Check sheet for the drawn part. Datum: minimum x, y, z corner. Units: mm. A direction names the side the tool comes from. Coordinates: 2 decimals unless noted, no trailing zeros. Write each loop counter-clockwise with the first axis right and the second up, starting at its lowest first coordinate (ties: lowest second). Pieces come first, ordered by that corner, then holes. Notation, with made-up numbers: (9, -39.5) -> (18, -39.5) arc R28 ccw to (18, -18.5) -> close; hole circle Ø4 at (29.25, 88). An arc over 180 degrees is marked (long way). Answer in a Markdown table with one row per item.
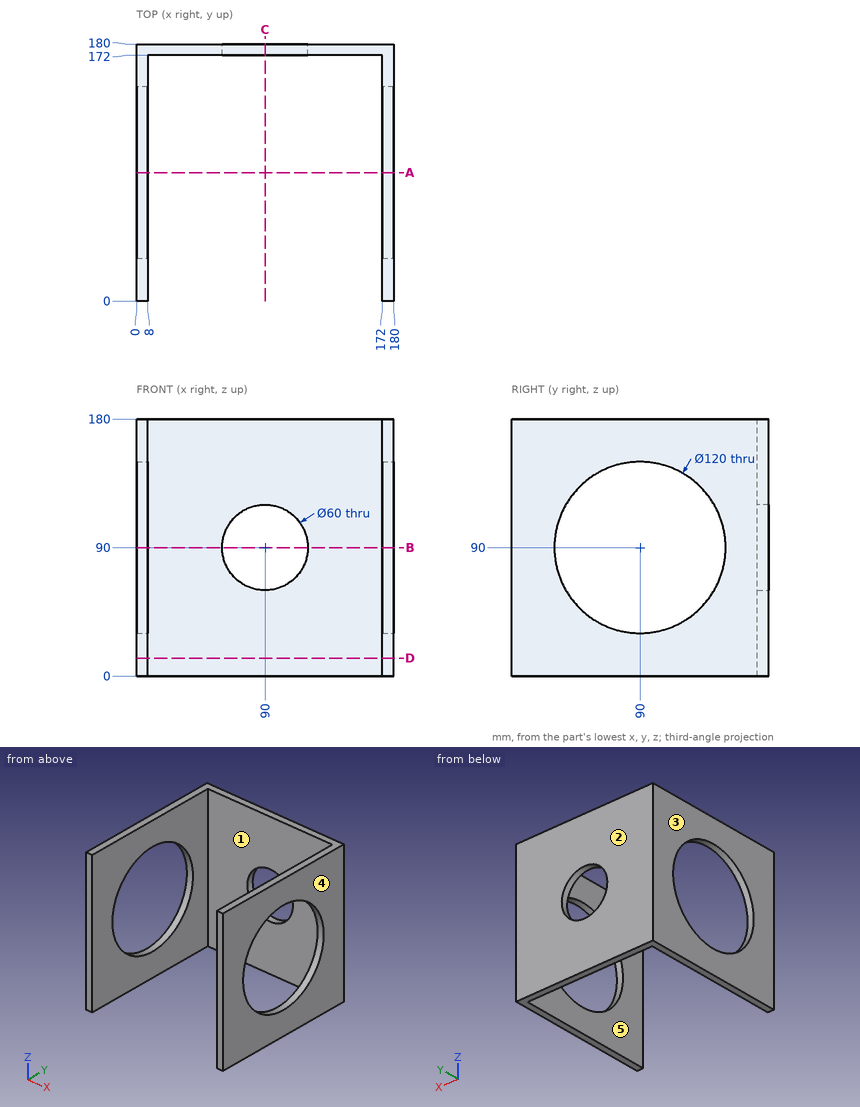
1. Sectioned sample at C-C, the plane x = 90. Record the cut outline in (y, z), and give its area (3 significant figures).
Findings below:
| item | result |
|---|---|
| outline | (172, 0) -> (180, 0) -> (180, 60) -> (172, 60) -> close; (172, 120) -> (180, 120) -> (180, 180) -> (172, 180) -> close |
| area | 960 mm² |
2. Material ranges on probe 1 along Z at (x, y) = (3, 90); probe 2 along X at (y, z) = (10.5, 97.5); probe 3 along Y at (x, z) = (34, 145.5), recorded low to high. Write a range as from..to.
Findings below:
| item | result |
|---|---|
| probe 1 | z = 0..30, 150..180 |
| probe 2 | x = 0..8, 172..180 |
| probe 3 | y = 172..180 |
3. Go/stop test with a flat-tipped pin: pin 1 (2 mm diameter, centred on x = 141, z = 111, fed in from -Y). Record where the tip stops, or that it passes through.
Findings below:
| item | result |
|---|---|
| pin 1 | stops at y = 172 |
4. Access from +Z, -Z, +X, -X, +Y, -Y to the whole of each face (thin tool, end or side, straight path). Record for the marked faces 1 and 2.
Findings below:
| item | result |
|---|---|
| face 1 | +Z, -Z, -Y |
| face 2 | +Z, -Z, +X, -X, +Y |
5. Sectioned sample at D-D, the plane z = 12.5. Record the cut outline in (x, y).
Findings below:
| item | result |
|---|---|
| outline | (0, 0) -> (8, 0) -> (8, 172) -> (172, 172) -> (172, 0) -> (180, 0) -> (180, 180) -> (0, 180) -> close |
6. Release check for a two-part mould opening along X. For the marked faces 3, 4 and 5 record: released by +X, released by -X, zero draft, split by the parting line, or undercut.
Findings below:
| item | result |
|---|---|
| face 3 | released by -X |
| face 4 | released by +X |
| face 5 | undercut |
7. Sectioned sample at A-A, the plane y = 90. Record the cut outline in (x, z), and give its area (3 significant figures).
Findings below:
| item | result |
|---|---|
| outline | (0, 0) -> (8, 0) -> (8, 30) -> (0, 30) -> close; (0, 150) -> (8, 150) -> (8, 180) -> (0, 180) -> close; (172, 0) -> (180, 0) -> (180, 30) -> (172, 30) -> close; (172, 150) -> (180, 150) -> (180, 180) -> (172, 180) -> close |
| area | 960 mm² |
8. Sectioned sample at B-B, the plane z = 90. Record the cut outline in (x, y), and give its area (3 significant figures).
Findings below:
| item | result |
|---|---|
| outline | (0, 0) -> (8, 0) -> (8, 30) -> (0, 30) -> close; (0, 150) -> (8, 150) -> (8, 172) -> (60, 172) -> (60, 180) -> (0, 180) -> close; (120, 172) -> (172, 172) -> (172, 150) -> (180, 150) -> (180, 180) -> (120, 180) -> close; (172, 0) -> (180, 0) -> (180, 30) -> (172, 30) -> close |
| area | 1,790 mm² |
